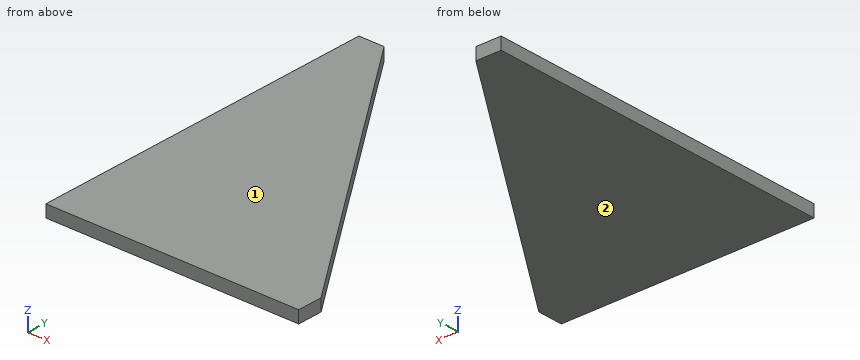
Autodesk Inventor part; units mm, degrees
ref_plane "YZ Plane" through (0, 0, 0) normal (1, 0, 0) x (0, 1, 0)
ref_plane "XZ Plane" through (0, 0, 0) normal (0, 1, 0) x (-1, 0, 0)
ref_plane "XY Plane" through (0, 0, 0) normal (0, 0, 1) x (1, 0, 0)
sketch "Sketch1" plane through (0, 0, 0) normal (0, 0, 1) x (1, 0, 0)
  line L0 (0, 0) -> (0, 88.9)
  line L1 (0, 88.9) -> (6.35, 88.9)
  line L2 (6.35, 88.9) -> (63.5, 6.35)
  line L3 (63.5, 6.35) -> (63.5, 0)
  line L4 (63.5, 0) -> (0, 0)
  dimension "d0" = 88.9
  dimension "d1" = 63.5
  dimension "d2" = 6.35
extrude "Extrusion1" add sketch "Sketch1" along normal mid plane 3.048
properties part number "A1-18002-100-52 Tube stop" material "Steel, Mild"
For this review, take the finished solid that the model builds, in its own axes (mm). Face numbers are marked on the shaded views. Give positions to 0.01 mm unless a question says otherwise; leave off trailing zeros. Write each loop counter-clockwise with the first axis right and the second up, starting at its lowest first coordinate (ties: lowest second). Pieces come first, ordered by that corner, then holes. Notation, with made-up numbers: M 54.5,-6.75 L 100.5,-6.75 A26 cw 100.5,26.25 Z; hole C 35.5,-28.75 d5. An arc over 180 degrees is marked long. Answer as CSV lines item,"result".
1. Consider section A-A, the plane z = 0.1. Write out the cut boundary in (x, y).
Findings:
outline,"M 0,0 L 63.5,0 L 63.5,6.35 L 6.35,88.9 L 0,88.9 Z"
2. Draft analysis for pull direction Z (two halves, no side actions). For the marked faces 1 and 2, state which applies: +Z half, -Z half, draft (parallel to the pull), parting line (faces both ways), or undercut.
Findings:
face 1,"+Z half"
face 2,"-Z half"
3. Wall thickness on line 1 (X direction, y = 26, z = 0.8); line 2 (Y direction, x = 18, z = -0.6); line 3 (Y direction, x = 26.5, z = -0.4): over which ranges is each line inside the solid? List them lowest first.
Findings:
line 1,"x = 0 to 49.9"
line 2,"y = 0 to 72.07"
line 3,"y = 0 to 59.79"
4. For pin 1 (1 mm diameter, centred on y = 38.5, z = 1, fed in from +X), flat-tipped, find the tip position at first contact; note if it passes through.
Findings:
pin 1,"stops at x = 41.59"
5. Consider section B-B, the plane x = 14. Write out the cut boundary in (y, z).
Findings:
outline,"M 0,-1.52 L 77.85,-1.52 L 77.85,1.52 L 0,1.52 Z"
6. Consider section C-C, the plane y = 10. Write out the cut boundary in (x, z), then the cut area to 3 significant figures.
Findings:
outline,"M 0,-1.52 L 60.97,-1.52 L 60.97,1.52 L 0,1.52 Z"
area,"186 mm2"
